from build123d import *

# Parameters (mm, degrees)
PAD_DEPTH       = 28.7
SKETCH001_R     = 1.75
POCKET_DEPTH    = 4.001
SKETCH002_W     = 1.75
SKETCH002_H     = 1.5
POCKET001_DEPTH = 134.001


with BuildPart() as part:
    # Sketch → Pad (new body)
    with BuildSketch(Plane.XZ):
        Polygon((-67, 0), (-35, 0), (-35, -32), (35, -32), (35, 0), (67, 0), (67, -4), (37, -4), (37, -34), (-37, -34), (-37, -4), (-67, -4), align=None)
    extrude(amount=PAD_DEPTH)

    # Sketch001 (on Face7 of Pad) → Pocket (cut, through all)
    with BuildSketch(Plane(origin=(0, 0, -4), x_dir=(1, 0, 0), z_dir=(0, 0, -1))):
        with Locations((-52, 14.35)):
            Circle(SKETCH001_R)
        with Locations((52, 14.35)):
            Circle(SKETCH001_R)
    extrude(amount=-POCKET_DEPTH, mode=Mode.SUBTRACT)

    # Sketch002 (on Face11 of Pocket) → Pocket001 (cut, through all)
    with BuildSketch(Plane(origin=(67, 0, 0), x_dir=(0, 0, 1), z_dir=(1, 0, 0))):
        with Locations((-1.875, 27.95)):
            Rectangle(SKETCH002_W, SKETCH002_H)
        with Locations((-1.875, 0.75)):
            Rectangle(SKETCH002_W, SKETCH002_H)
    extrude(amount=-POCKET001_DEPTH, mode=Mode.SUBTRACT)


solid = part.part
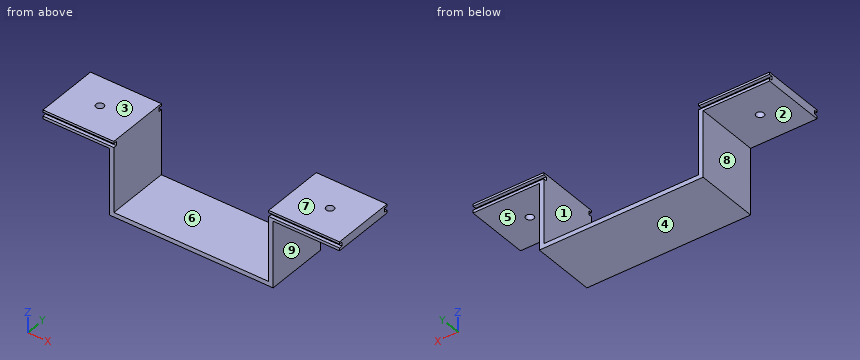
Part model, mm, in its own coordinate system. Face numbers are marked on the shaded views. A direction names the side the tool comes from. Coordinates: 2 decimals unless noted, no trailing zeros. Order: outer loops, then holes, each group sorted by start corner. A loop starts at its lowest first (then second) coordinate and runs counter-clockwise, first axis right, second up. Notation, with made-up numbers: (-8.75, 65.5) - (40.25, 65.5) arc R16 ccw to (40.25, 92.5) - close; hole circle Ø9 at (25, 22.5). An arc over 180 degrees is marked (long way). Use CSV: the item, a comma, the result in double quotes.
Item 1: Probe probe 1 along X at (y, z) = (-14.35, -0.9); probe 2 along X at (y, z) = (-13, -17.5); probe 3 along Y at (x, z) = (52, -1.7). List the from-to ranges inside material, lowest first.
Solved:
probe 1,"x = -67 to -53.75, -50.25 to -35, 35 to 50.25, 53.75 to 67"
probe 2,"x = -37 to -35, 35 to 37"
probe 3,"y = -27.2 to -16.1, -12.6 to -1.5"
Item 2: Saw through at A-A on x = 52. Give the cut face in (y, z).
Solved:
outline,"(-28.7, -4) - (-16.1, -4) - (-16.1, 0) - (-28.7, 0) - (-28.7, -1) - (-27.2, -1) - (-27.2, -2.75) - (-28.7, -2.75) - close; (-12.6, -4) - (0, -4) - (0, -2.75) - (-1.5, -2.75) - (-1.5, -1) - (0, -1) - (0, 0) - (-12.6, 0) - close"
Item 3: Mould opens along X. For the marked faces 6, 7, 8 and 9 say: +X half, -X half, draft (parallel to the pull), parting line (faces both ways), or undercut.
Solved:
face 6,"undercut"
face 7,"draft"
face 8,"-X half"
face 9,"+X half"
Item 4: Saw through at C-C on y = -14.35. Give the cut face in (x, z).
Solved:
outline,"(-67, -4) - (-53.75, -4) - (-53.75, 0) - (-67, 0) - close; (-50.25, -4) - (-37, -4) - (-37, -34) - (37, -34) - (37, -4) - (50.25, -4) - (50.25, 0) - (35, 0) - (35, -32) - (-35, -32) - (-35, 0) - (-50.25, 0) - close; (53.75, -4) - (67, -4) - (67, 0) - (53.75, 0) - close"
Item 5: Saw through at B-B on z = -29. Give the cut face in (x, y).
Solved:
outline,"(-37, -28.7) - (-35, -28.7) - (-35, 0) - (-37, 0) - close; (35, -28.7) - (37, -28.7) - (37, 0) - (35, 0) - close"
Item 6: 3-axis set-ups, long thin cutter, end or side, ignore diameter. For the marked faces 1, 2, 3, 4 and 5: which of +Z, -Z, +X, -X, +Y, -Y reach the whole face in a straight line?
Solved:
face 1,"+Z, +Y, -Y"
face 2,"-Z, -X, +Y, -Y"
face 3,"+Z, +X, -X, +Y, -Y"
face 4,"-Z, +X, -X, +Y, -Y"
face 5,"-Z, +X, +Y, -Y"
Item 7: Drop flat-ended pins along their axis: P1, Ø4, axis at x = -52, y = -14.35, coming from the -Z side; P2, Ø12, axis at x = -44.5, z = -17, coming from the +Y side; P3, Ø3, axis at y = -16.5, z = -24, coming from the -X side; P4, Ø3, axis at x = 1, y = -3, coming from the +Z side. Give the stop position or say it passes through.
Solved:
P1,"stops at z = -4"
P2,"passes through"
P3,"stops at x = -37"
P4,"stops at z = -32"
Item 8: Saw through at D-D on y = -25.5. Give the cut face in (x, z), and give its area (3 significant figures).
Solved:
outline,"(-67, -4) - (-37, -4) - (-37, -34) - (37, -34) - (37, -4) - (67, -4) - (67, 0) - (35, 0) - (35, -32) - (-35, -32) - (-35, 0) - (-67, 0) - close"
area,"516 mm²"
